Geometry check sheet. Reference: the model listing, model coordinates, mm. A direction names the side the tool comes from. Coordinates: 2 decimals unless noted, no trailing zeros. One line per item, written item: value. Start each with the question number.
1) Go/stop test with flat-tipped pins: P1, Ø5, axis at y = 9, z = 11, coming from the +X side; P2, Ø5, axis at x = 8.5, y = 3.5, coming from the +Z side; P3, Ø1, axis at x = 24.5, y = 5.5, coming from the -Z side. Record where each tip stops, or that it passes through.
2) Thickness scan on L1, parallel to Z at x = 3, y = 9; L2, parallel to Z at x = 17.5, y = 9.5; L3, parallel to Y at x = 6.75, z = 113.5. Record the ranges inside material, lowest first. Write a range as from..to.
3) Sectioned sample at A-A, the plane y = 9. State how many separate pieces and enclosed holes the cut face has, then the cut area to 3 significant figures.
4) Access from +Z, -Z, +X, -X, +Y, -Y to the whole of each face (thin tool, end or side, straight path). Record for faces 4 (the cylindrical face through (15.838, 2.979, 88.834)), 5 (the flat face through (4.5, 7, 7)), 6 (the flat face through (14, 4.5, 30)).
5) Draft check along X on faces 1 (the flat face through (15, 1.5, 58)), 2 (the flat face through (15.2, 5.3, 105.3)), 3 (the cylindrical face through (16.222, 2.979, 29.234)). Enter one of: pulls with the +X half, pulls with the -X half, needs draft (parallel to the pull), parting line crosses it, or undercut.
```python
from build123d import *

# Parameters (mm, degrees)
EXTRU_MINCE1_DEPTH      = 118
ESQUISSE2_R             = 2.5
ENL_V_MAT_EXTRU_1_DEPTH = 4
ESQUISSE3_R             = 1.5
ENL_V_MAT_EXTRU_2_DEPTH = 4
CHANFREIN1_SIZE         = 25
BOSS_EXTRU_1_DEPTH      = 118
ESQUISSE5_R             = 2.5
ENL_V_MAT_EXTRU_3_DEPTH = 122.820564897
ESQUISSE6_R             = 1.5
ENL_V_MAT_EXTRU_4_DEPTH = 123.149498698
ENL_V_START             = -3
ESQUISSE8_R             = 5
ENL_V_MAT_EXTRU_5_DEPTH = 119.820564897
ENL_V_MAT_EXTRU_6_DEPTH = 119.9682337
ENL_V_MAT_EXTRU_6_TAPER = -2


with BuildPart() as part:
    # Esquisse1 → Extru.-Mince1 (new body)
    with BuildSketch(Plane.XY):
        Polygon((0, 15.5), (0, 0), (27.5, 0), (27.5, 1.5), (1.5, 1.5), (1.5, 15.5), align=None)
    extrude(amount=EXTRU_MINCE1_DEPTH)

    # Esquisse2 → Enlèv. mat.-Extru.1 (cut)
    with BuildSketch(Plane.ZY):
        with Locations(Location((9, 9, 0), (0, 0, 270))):
            Circle(ESQUISSE2_R)
        with Locations(Location((109, 9, 0), (0, 0, 90))):
            Circle(ESQUISSE2_R)
    extrude(amount=-ENL_V_MAT_EXTRU_1_DEPTH, mode=Mode.SUBTRACT)

    # Esquisse3 → Enlèv. mat.-Extru.2 (cut)
    with BuildSketch(Plane.XZ):
        with Locations(Location((15.771636742, 30.664864187, 0), (0, 0, 270))):
            Circle(ESQUISSE3_R)
        with Locations(Location((15.771636742, 87.335135813, 0), (0, 0, 90))):
            Circle(ESQUISSE3_R)
    extrude(amount=-ENL_V_MAT_EXTRU_2_DEPTH, mode=Mode.SUBTRACT)

    # Chanfrein1
    chanfrein1_edges = [part.edges().sort_by_distance(p)[0] for p in [
        (27.5, 0.75, 0),
        (27.5, 0.75, 118),
    ]]
    chamfer(chanfrein1_edges, length=CHANFREIN1_SIZE)


with BuildPart() as body_2:
    # Esquisse4 → Boss.-Extru.1 (new body)
    with BuildSketch(Plane(origin=(0, 0, 0), x_dir=(-1, 0, 0), z_dir=(0, 0, -1))):
        with BuildLine():
            Line((-27.5, 1.5), (-1.5, 1.5))
            Line((-1.5, 1.5), (-1.5, 15.5))
            add(Edge.make_bspline(
                [(-1.5, 15.5), (-27.5, 15.5), (-27.5, 1.5)],
                knots=[4.71238898, 4.71238898, 4.71238898, 6.283185307, 6.283185307, 6.283185307], degree=2, weights=[1, 0.707106781, 1]))
        make_face()
    extrude(amount=-BOSS_EXTRU_1_DEPTH)

    # Esquisse5 → Enlèv. mat.-Extru.3 (cut, through all)
    with BuildSketch(Plane.ZY.offset(-1.5)):
        with Locations(Location((109, 9, 0), (0, 0, 270))):
            Circle(ESQUISSE5_R)
        with Locations(Location((9, 9, 0), (0, 0, 270))):
            Circle(ESQUISSE5_R)
    extrude(amount=-ENL_V_MAT_EXTRU_3_DEPTH, mode=Mode.SUBTRACT)

    # Esquisse6 → Enlèv. mat.-Extru.4 (cut, through all)
    with BuildSketch(Plane.XZ):
        with Locations(Location((15.771636742, 87.335135813, 0), (0, 0, 270))):
            Circle(ESQUISSE6_R)
        with Locations(Location((15.771636742, 30.664864187, 0), (0, 0, 270))):
            Circle(ESQUISSE6_R)
        Polygon((27.5, 93), (2.5, 118), (27.5, 118), align=None)
        Polygon((2.5, 0), (27.5, 25), (27.5, 0), align=None)
    extrude(amount=-ENL_V_MAT_EXTRU_4_DEPTH, mode=Mode.SUBTRACT)

    # Esquisse8 → Enlèv. mat.-Extru.5 (cut, through all)
    with BuildSketch(Plane.ZY.offset(-1.5).offset(ENL_V_START)):
        with Locations(Location((9, 9, 0), (0, 0, 270))):
            Circle(ESQUISSE8_R)
        with Locations(Location((109, 9, 0), (0, 0, 270))):
            Circle(ESQUISSE8_R)
    extrude(amount=-ENL_V_MAT_EXTRU_5_DEPTH, mode=Mode.SUBTRACT)

    # Esquisse9 → Enlèv. mat.-Extru.6 (cut, through all)
    with BuildSketch(Plane.XZ.offset(-1.5).offset(ENL_V_START)):
        Polygon((19.062533276, 87.335135813), (17.417085009, 90.185135813), (14.126188475, 90.185135813), (12.480740208, 87.335135813), (14.126188475, 84.485135813), (17.417085009, 84.485135813), align=None)
        Polygon((17.417085009, 33.514864187), (14.126188475, 33.514864187), (12.480740208, 30.664864187), (14.126188475, 27.814864187), (17.417085009, 27.814864187), (19.062533276, 30.664864187), align=None)
    extrude(amount=-ENL_V_MAT_EXTRU_6_DEPTH, taper=ENL_V_MAT_EXTRU_6_TAPER, mode=Mode.SUBTRACT)


solid = body_2.part
```
Final values:
1. P1: stops at x = 4.5
1. P2: stops at z = 114.5
1. P3: stops at z = 21.5
2. L1: z = 0.5..6.5, 11.5..106.5, 111.5..117.5
2. L2: z = 15..27.64, 33.69..84.31, 90.36..103
2. L3: y = 1.5..6.82, 11.18..15.21
3. separate pieces: 3
3. enclosed holes: 2
3. area: 1,920 mm^2
4. face 4: +Y, -Y
4. face 5: +X
4. face 6: +Y
5. face 1: needs draft
5. face 2: pulls with the +X half
5. face 3: undercut
